Source: CAD feature listing. Evaluate the final solid. Frame: model axes, mm. Round coordinates to 2 decimals unless told otherwise and drop trailing zeros. Order: outer loops, then holes, each group sorted by start corner. A loop starts at its lowest first (then second) coordinate and runs counter-clockwise, first axis right, second up. Notation, with made-up numbers: (64, 21.5) -> (109, 21.5) arc R22 ccw to (109, 45.5) -> close; hole circle Ø1 at (57, 81). An arc over 180 degrees is marked (long way). Write item = value, one per line. Start each with the question number.
(1) Cut plane C-C on z = 465.5. Return the cut outline in (x, y), then the cut area to 3 significant figures.
(2) Cut plane B-B on z = 286. Return the cut outline in (x, y).
(3) Cut plane A-A on x = 14. Return the cut outline in (y, z), then the cut area to 3 significant figures.
(4) Ray query, line 1 (Y direction, x = -8.5, z = 64.5); line 2 (X direction, y = -13, z = 52); line 3 (Y direction, x = 23, z = 451.5). Return the intervals inside material, ascending.
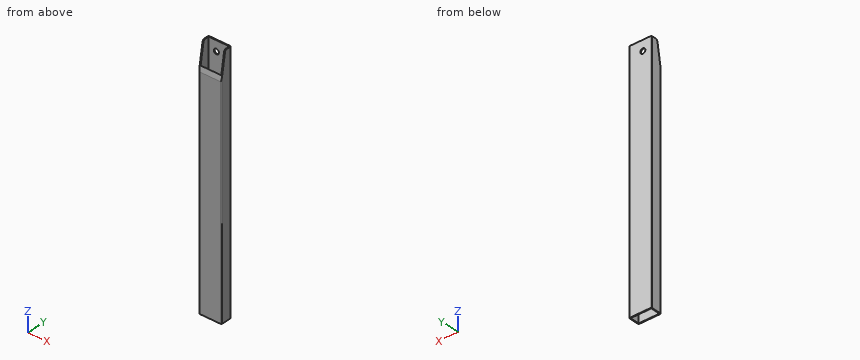
Autodesk Inventor part; units mm, degrees
ref_plane "YZ Plane" through (0, 0, 0) normal (1, 0, 0) x (0, 1, 0)
ref_plane "XZ Plane" through (0, 0, 0) normal (0, 1, 0) x (-1, 0, 0)
ref_plane "XY Plane" through (0, 0, 0) normal (0, 0, 1) x (1, 0, 0)
sketch "Sketch1" plane through (0, 0, 0) normal (0, 0, 1) x (1, 0, 0)
  line L0 (-50, 25) -> (50, 25)
  line L1 (50, 25) -> (50, -25)
  line L2 (50, -25) -> (-50, -25)
  line L3 (-50, -25) -> (-50, 25)
  line L4 (-50, 25) -> (50, -25) construction
  line L5 (50, 25) -> (-50, -25) construction
  point P0 (0, 0)
  dimension "d0" = 100
  dimension "d1" = 50
extrude "Extrusion1" add sketch "Sketch1" along normal mid plane 1100
fillet "Fillet1" radius 4 4 edges at (50, -25, 0) (50, 25, 0) (-50, -25, 0) (-50, 25, 0)
shell "Shell1" thickness 4 removed faces 2 at (-15.3333, -8.3333, 550) at (-15.3333, -8.3333, -550)
sketch "Sketch2" plane through (-46, 25, 550) normal (0, 1, 0) x (1, 0, 0)
  circle A0 centre (34.3509, 45.5772) radius 11.25
  point P0 (46, 550)
extrude "Extrusion2" cut sketch "Sketch2" against normal through all
sketch "Sketch3" plane through (50, -21, 550) normal (1, 0, 0) x (0, 0, -1)
  line L0 (0, -4) -> (1100, -4)
  line L1 (0, 42) -> (0, 0)
  line L2 (0, 16) -> (120, -4)
  line L3 (0, -11.4428) -> (0, 16)
  line L4 (120, -4) -> (120, -11.4428)
  line L5 (120, -11.4428) -> (0, -11.4428)
  point P0 (550, 21)
  dimension "d8" = 120
  dimension "d9" = 20
extrude "Extrusion3" cut sketch "Sketch3" against normal blind 1100
fillet "Fillet2" radius 10 2 edges at (48, -5, 550) (-48, -5, 550)
sketch "Sketch4" plane through (-46, 25, 550) normal (0, 1, 0) x (1, 0, 0)
  line L0 (90.5966, 11.6068) -> (90.5966, 2.7213) construction
  line L1 (90.5966, 2.7213) -> (86.2672, 2.7213) construction
  line L2 (86.2672, 2.7213) -> (86.2672, 11.6068) construction
  line L3 (86.2672, 11.6068) -> (90.5966, 11.6068) construction
  point P0 (46, 550)
properties part number "MC02-1"
Evaluation:
q1.outline = (-50, -19.08) -> (-46, -19.08) -> (-46, 21) -> (46, 21) -> (46, -19.08) -> (50, -19.08) -> (50, 21) arc R4 ccw to (46, 25) -> (-46, 25) arc R4 ccw to (-50, 21) -> close
q1.area = 714 mm^2
q2.outline = (-50, -21) arc R4 ccw to (-46, -25) -> (46, -25) arc R4 ccw to (50, -21) -> (50, 21) arc R4 ccw to (46, 25) -> (-46, 25) arc R4 ccw to (-50, 21) -> close; hole (-46, -21) -> (46, -21) -> (46, 21) -> (-46, 21) -> close
q3.outline = (-25, -550) -> (-21, -550) -> (-21, 454) -> (-25, 430) -> close; (21, -550) -> (25, -550) -> (25, 550) -> (21, 550) -> close
q3.area = 8,370 mm^2
q4.line_1 = -25 to -21, 21 to 25
q4.line_2 = -50 to -46, 46 to 50
q4.line_3 = -21.42 to -21, 21 to 25
